Verification items for the finished model (mm, model axes). A direction names the side the tool comes from. Coordinates: 2 decimals unless noted, no trailing zeros. Order: outer loops, then holes, each group sorted by start corner. A loop starts at its lowest first (then second) coordinate and runs counter-clockwise, first axis right, second up. Notation, with made-up numbers: M 74.25,5.5 L 133.25,5.5 A21 ccw 133.25,10.5 Z; hole C 69,34.5 d11. An arc over 180 degrees is marked long. Write item = value, one per line.
```python
from build123d import *

# Parameters (mm, degrees)
BOSS_EXTRUDE1_DEPTH          = 1.5875
FILLET3_R                    = 8
FILLET4_R                    = 8
BOSS_EXTRUDE3_DEPTH          = 1.5875
EDGE_FLANGE1_STRIP_W         = 26.35
EDGE_FLANGE1_STRIP_H         = 1.5875
EDGE_FLANGE1_STRIP_CUT_DEPTH = 14
EDGE_FLANGE1_DEPTH           = 14
FILLET5_R                    = 10
FILLET9_R                    = 2


# Sheet-metal steps are written as plain solids
with BuildPart() as part:
    # Sketch3 → Boss-Extrude1 (new body)
    with BuildSketch(Plane.XY):
        Polygon((58.775, 33.228336454), (53.202823644, 29.668334894), (46.775, 25.561669788), (40.347176356, 29.668334894), (34.775, 33.228336454), (22.775, 25.561669788), (14.005335663, 31.164510892), (7.544664337, 21.052155774), (22.775, 11.321663546), (28.347176356, 14.881665106), (34.775, 18.988330212), (41.202823644, 14.881665106), (46.775, 11.321663546), (58.775, 18.988330212), (67.544664337, 13.385489108), (74.005335663, 23.497844226), align=None)
    extrude(amount=BOSS_EXTRUDE1_DEPTH)

    # Fillet3
    fillet3_edges = [part.edges().sort_by_distance(p)[0] for p in [
        (46.775, 11.321663546, 0.79375),
        (22.775, 11.321663546, 0.79375),
        (34.775, 33.228336454, 0.79375),
        (58.775, 33.228336454, 0.79375),
    ]]
    fillet(fillet3_edges, radius=FILLET3_R)

    # Fillet4
    fillet4_edges = [part.edges().sort_by_distance(p)[0] for p in [
        (34.775, 18.988330212, 0.79375),
        (22.775, 25.561669788, 0.79375),
        (46.775, 25.561669788, 0.79375),
        (58.775, 18.988330212, 0.79375),
    ]]
    fillet(fillet4_edges, radius=FILLET4_R)

    # Sketch5 → Boss-Extrude3 (add)
    with BuildSketch(Plane(origin=(0, 0, 0), x_dir=(-1, 0, 0), z_dir=(0, 0, -1))):
        Polygon((20.994664337, 31.164510892), (-14.005335663, 31.164510892), (-7.544664337, 21.052155774), (-13.629673718, 17.164510892), (20.994664337, 17.164510892), align=None)
    extrude(amount=-BOSS_EXTRUDE3_DEPTH)

    # Edge-Flange1 strip (across the edge) → Edge-Flange1 strip cut (cut)
    with BuildSketch(Plane(origin=(-20.994664337, 31.164510892, 1.5875), x_dir=(1, 0, 0), z_dir=(0, -1, 0))):
        with Locations((-1.5875, -0.79375)):
            Rectangle(EDGE_FLANGE1_STRIP_W, EDGE_FLANGE1_STRIP_H)
    extrude(amount=EDGE_FLANGE1_STRIP_CUT_DEPTH, mode=Mode.SUBTRACT)

    # Edge-Flange1 section (across the edge) → Edge-Flange1 (add)
    with BuildSketch(Plane(origin=(-20.994664337, 31.164510892, 1.5875), x_dir=(1, 0, 0), z_dir=(0, -1, 0))):
        with BuildLine():
            Line((0, 10), (0, 40.4125))
            Line((0, 40.4125), (1.5875, 40.4125))
            Line((1.5875, 40.4125), (1.5875, 10))
            ThreePointArc((1.5875, 10), (4.516432188, 2.928932188), (11.5875, 0))
            Line((11.5875, 0), (11.5875, -1.5875))
            ThreePointArc((11.5875, -1.5875), (3.393900173, 1.806400173), (0, 10))
        make_face()
    extrude(amount=EDGE_FLANGE1_DEPTH)

    # Fillet5
    fillet5_edges = [part.edges().sort_by_distance(p)[0] for p in [
        (14.005335663, 31.164510892, 0.79375),
        (13.629673718, 17.164510892, 0.79375),
    ]]
    fillet(fillet5_edges, radius=FILLET5_R)

    # Fillet9
    fillet9_edges = [part.edges().sort_by_distance(p)[0] for p in [
        (67.544664337, 13.385489108, 0.79375),
        (74.005335663, 23.497844226, 0.79375),
        (-20.200914337, 31.164510892, 42),
        (-20.200914337, 17.164510892, 42),
    ]]
    fillet(fillet9_edges, radius=FILLET9_R)


solid = part.part
```
Item 1: Sectioned sample at B-B, the plane z = 31.5. Enter the section's corners in (x, y).
Report:
outline = M -20.99,17.16 L -19.41,17.16 L -19.41,31.16 L -20.99,31.16 Z
Item 2: Release check for a two-part mould opening along X. For faces 4 (the cylindrical face through (73.2, 23.3, 0.8)), 5 (the cylindrical face through (34.839, 17.495, 0.805)), 6 (the flat face through (17.263, 14.843, 0.783)) record: pulls with the +X half, pulls with the -X half, needs draft (parallel to the pull), parting line crosses it, or undercut.
Report:
face_4 = pulls with the +X half
face_5 = undercut
face_6 = pulls with the -X half
Item 3: Gauge pin test, flat ends, axial feed: pin 1 (2 mm diameter, centred on x = 46, y = 19.5, fed in from +Z); pin 2 (9.5 mm diameter, centred on x = -12, z = 13.5, fed in from -Y); pin 3 (11 mm diameter, centred on y = 27.5, z = 22, fed in from +X). Record the tip position at first contact, or that the pin passes through.
Report:
pin_1 = 1.59
pin_2 = through
pin_3 = -19.41
Item 4: Sectioned sample at A-A, the plane y = 25.5. Enter the section's corners in (x, z) (1 decimal).
Report:
outline = M -21,11.6 A11.6 ccw -9.4,0 L 70.9,0 L 70.9,1.6 L -9.4,1.6 A10 cw -19.4,11.6 L -19.4,42 L -21,42 Z
Item 5: Tool access check on faces 1 (the flat face through (28.8, 29.41, 0.78)), 2 (the flat face through (-19.407, 24, 27)), 3 (the flat face through (-19, 31.165, 8)). Record the directions out of +Z, -Z, +X, -X, +Y, -Y that give a thin tool (end or side, any length) a straight path to the whole face; none if there is none.
Report:
face_1 = +Z, -Z, +Y
face_2 = +Z, +X, +Y, -Y
face_3 = +Z, -Z, -X, +Y
Item 6: Sectioned sample at C-C, the plane x = -8.5. Enter the section's corners in (y, z).
Report:
outline = M 17.16,0 L 31.16,0 L 31.16,1.59 L 17.16,1.59 Z
Item 7: Scan lines: L1, parallel to Z at x = 38, y = 26; L2, parallel to X at y = 28.5, z = 12.5; L3, parallel to X at y = 22, z = 8.5. Record each from-to range of solid material in increasing order. Write a range as from..to.
Report:
L1 = 0..1.59
L2 = -20.99..-19.41
L3 = -20.58..-18.92
